Autodesk Inventor part; units mm, degrees
ref_plane "YZ Plane" through (0, 0, 0) normal (1, 0, 0) x (0, 1, 0)
ref_plane "XZ Plane" through (0, 0, 0) normal (0, 1, 0) x (-1, 0, 0)
ref_plane "XY Plane" through (0, 0, 0) normal (0, 0, 1) x (1, 0, 0)
sketch "Эскиз1" plane through (0, 0, 0) normal (0, 0, 1) x (1, 0, 0)
  line L0 (0, 0) -> (0, 57.7087)
  line L1 (0, 0) -> (87.3611, 0) construction
  line L2 (21.4984, 0) -> (24.079, 64)
  line L3 (24.079, 64) -> (27.5, 64)
  line L4 (27.5, 64) -> (27.5, 62)
  line L5 (27.5, 62) -> (26, 62)
  line L6 (26, 62) -> (23.5, 0)
  line L7 (21.4984, 0) -> (23.5, 0)
  line L8 (23.5, 0) -> (0, 0)
  line L9 (0, 0) -> (0, 2)
  line L10 (0, 2) -> (21.579, 2)
  dimension "d0" = 47
  dimension "d1" = 52
  dimension "d2" = 55
  dimension "d3" = 62
  dimension "d4" = 2
  dimension "d5" = 2
  dimension "d8" = 2
revolve "Вращение1" add sketch "Эскиз1" angle 360 about axis through (0, 0, 0) along (0, 1, 0)
fillet "Сопряжение1" radius 2 1 edges at (-23.5, 0, 0)
equation "\"d8\" = d4"
properties part number "Стакан_В2"
The listing builds one solid part. Answer for the finished solid, in the listing's coordinates (mm). A direction names the side the tool comes from. Give positions to 0.01 mm unless a question says otherwise; leave off trailing zeros. Write each loop counter-clockwise with the first axis right and the second up, starting at its lowest first coordinate (ties: lowest second). Pieces come first, ordered by that corner, then holes. Notation, with made-up numbers: (17.25, 3.25) -> (69.25, 3.25) arc R13 ccw to (69.25, 21.25) -> close; hole circle Ø4 at (65, 80.5). An arc over 180 degrees is marked (long way). Use a Markdown table: item, result.
(1) Section A-A, the plane z = 0 is taken. Determine the outline of the cut face in (x, y), then the cut area to 3 significant figures.
Return value:
| item | result |
|---|---|
| outline | (-27.5, 62) -> (-26, 62) -> (-23.58, 1.92) arc R2 ccw to (-21.58, 0) -> (21.58, 0) arc R2 ccw to (23.58, 1.92) -> (26, 62) -> (27.5, 62) -> (27.5, 64) -> (24.08, 64) -> (21.58, 2) -> (-21.58, 2) -> (-24.08, 64) -> (-27.5, 64) -> close |
| area | 347 mm2 |
(2) For faces 4 (the conical face through (-2.974, 33.434, -22.652)), 5 (the flat face through (10.1, 62, 24.3)), determine the directions among +Z, -Z, +X, -X, +Y, -Y from which every point of the face is accessible in a straight line to the end or side of a thin tool.
Return value:
| item | result |
|---|---|
| face 4 | +Y |
| face 5 | -Y |
(3) Flat-ended cylindrical pins translate along their axes: P1, Ø1, axis at x = -2, y = 57, coming from the -Z side; P2, Ø1.5, axis at y = 52, z = 13, coming from the -X side; P3, Ø1.5, axis at y = 14, z = 20, coming from the +X side. Find the tip coordinate at first contact, or state that the pin passes through.
Return value:
| item | result |
|---|---|
| P1 | z = -25.76 |
| P2 | x = -22.48 |
| P3 | x = 14.44 |
(4) Section D-D, the plane y = 28 is taken. Determine the outline of the cut face in (x, z).
Return value:
| item | result |
|---|---|
| outline | circle Ø49.26 at (0, 0); hole circle Ø45.25 at (0, 0) |
(5) Determine the mould class of faces 1 (the flat face through (0, 0, 0)), 2 (the flat face through (0, 2, 0)), 3 (the cylindrical face through (-5.961, 62.986, -26.846)) for opening direction Z: released by +Z, released by -Z, zero draft, split by the parting line, or undercut.
Return value:
| item | result |
|---|---|
| face 1 | zero draft |
| face 2 | undercut |
| face 3 | split by the parting line |
(6) Find the intervals of material crossed by probe 1 along Y at (x, z) = (-11.5, -17.5); probe 2 along X at (y, z) = (40, -14); probe 3 along Z at (x, y) = (-21.5, 57.5), in increasing order. Write a range as from..to.
Return value:
| item | result |
|---|---|
| probe 1 | 0..2 |
| probe 2 | -20.85..-18.39, 18.39..20.85 |
| probe 3 | -14.3..-10.25, 10.25..14.3 |
(7) Section B-B, the plane x = 0 is taken. Determine the outline of the cut face in (y, z).
Return value:
| item | result |
|---|---|
| outline | (0, -21.58) arc R2 ccw to (1.92, -23.58) -> (62, -26) -> (62, -27.5) -> (64, -27.5) -> (64, -24.08) -> (2, -21.58) -> (2, 21.58) -> (64, 24.08) -> (64, 27.5) -> (62, 27.5) -> (62, 26) -> (1.92, 23.58) arc R2 ccw to (0, 21.58) -> close |
(8) Section C-C, the plane y = 8 is taken. Determine the outline of the cut face in (x, z), then the cut area to 3 significant figures.
Return value:
| item | result |
|---|---|
| outline | circle Ø47.65 at (0, 0); hole circle Ø43.64 at (0, 0) |
| area | 287 mm2 |
